Part model, mm, in its own coordinate system. A direction names the side the tool comes from. Give positions to 0.01 mm unless a question says otherwise; leave off trailing zeros. Order: outer loops, then holes, each group sorted by start corner. A loop starts at its lowest first (then second) coordinate and runs counter-clockwise, first axis right, second up. Notation, with made-up numbers: M -9,-24 L 12,-24 A13 cw 12,-13 Z; hole C 31.5,15.25 d2. An arc over 180 degrees is marked long. One line per question, with ' | ' between items.
```python
from build123d import *

# Parameters (mm, degrees)
EXTRUDE_1_DEPTH     = 40
SKETCH_2_R          = 2.5
CUT_EXTRUDE_1_DEPTH = 12
SKETCH_3_R          = 3
EXTRUDE_2_DEPTH     = 8
CHAMFER_1_SIZE      = 0.2


with BuildPart() as part:
    # 草图1 → 凸台-拉伸1 (new body)
    with BuildSketch(Plane(origin=(0, 0, 0), x_dir=(0, 0, -1), z_dir=(1, 0, 0))):
        Polygon((4.618802154, 0), (2.309401077, 4), (-2.309401077, 4), (-4.618802154, 0), (-2.309401077, -4), (2.309401077, -4), align=None)
    extrude(amount=EXTRUDE_1_DEPTH)

    # 草图2 → 切除-拉伸1 (cut)
    with BuildSketch(Plane(origin=(40, 0, 0), x_dir=(0, 0, -1), z_dir=(1, 0, 0))):
        Circle(SKETCH_2_R)
    extrude(amount=-CUT_EXTRUDE_1_DEPTH, mode=Mode.SUBTRACT)

    # 草图3 → 凸台-拉伸2 (add)
    with BuildSketch(Plane.ZY):
        Circle(SKETCH_3_R)
    extrude(amount=EXTRUDE_2_DEPTH)

    # 倒角1
    chamfer_1_edges = [part.edges().sort_by_distance(p)[0] for p in [
        (-8, 0, -3),
    ]]
    chamfer(chamfer_1_edges, length=CHAMFER_1_SIZE)


solid = part.part
```
1. Slice it at B-B on x = 26.5. Give the cut face in (y, z), then the cut area to 3 significant figures.
Worked out:
outline: M -4,-2.31 L 0,-4.62 L 4,-2.31 L 4,2.31 L 0,4.62 L -4,2.31 Z | area: 55.4 mm2
2. Probe L1, parallel to Y at x = 32, z = 0; L2, parallel to X at y = 1.5, z = -1.5; L3, parallel to X at y = -0.5, z = -3.75. List the from-to ranges inside material, lowest first. Write a range as from..to.
Worked out:
L1: y = -4..-2.5, 2.5..4 | L2: x = -8..28 | L3: x = 0..40
3. Mould opens along Z. For faces 1 (the flat face through (40, 2, -2)), 2 (the cylindrical face through (34.08, -2.44, 0.54)), 3 (the flat face through (19.72, 1.97, -3.48)) say: released by +Z, released by -Z, zero draft, split by the parting line, or undercut.
Worked out:
face 1: zero draft | face 2: undercut | face 3: released by -Z
4. Slice it at C-C on z = 3.75. Give the cut face in (x, y), then the cut area to 3 significant figures.
Worked out:
outline: M 0,-1.5 L 40,-1.5 L 40,1.5 L 0,1.5 Z | area: 120 mm2
5. Slice it at A-A on z = 0. Give the cut face in (x, y), then the cut area to 3 significant figures.
Worked out:
outline: M -8,-2.8 L -7.8,-3 L 0,-3 L 0,-4 L 40,-4 L 40,-2.5 L 28,-2.5 L 28,2.5 L 40,2.5 L 40,4 L 0,4 L 0,3 L -7.8,3 L -8,2.8 Z | area: 308 mm2
6. Tool access for faces 4 (the flat face through (19.72, -2.028, -3.448)), 5 (the flat face through (28, 0, 0)), 6 (the flat face through (0, 1, -3)): list every direction of +Z, -Z, +X, -X, +Y, -Y with a clear straight run to the whole face (end or side of a thin tool).
Worked out:
face 4: -Z, +X, -X, -Y | face 5: +X | face 6: -X
7. Drop flat-ended pins along their axis: pin 1 (1.5 mm diameter, centred on y = 0.5, z = 0.5, fed in from +X); pin 2 (3 mm diameter, centred on x = 10.5, y = -2, fed in from -Z); pin 3 (1 mm diameter, centred on x = 2, y = 3, fed in from +Z). Give the stop position or say it passes through.
Worked out:
pin 1: stops at x = 28 | pin 2: stops at z = -4.33 | pin 3: stops at z = 3.18
